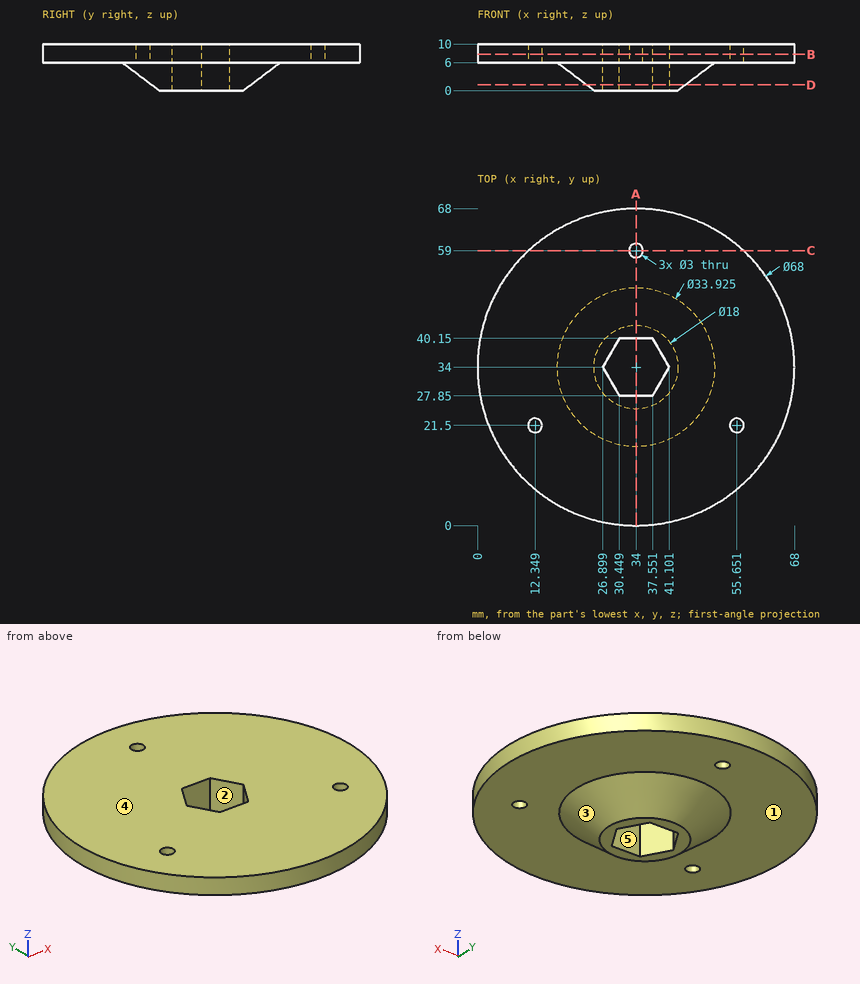
Could you check a few things on this drawing? It's one solid part, dimensions in mm from its lowest x, y, z. A direction names the side the tool comes from. Coordinates: 2 decimals unless noted, no trailing zeros. Order: outer loops, then holes, each group sorted by start corner. A loop starts at its lowest first (then second) coordinate and runs counter-clockwise, first axis right, second up. Notation, with made-up numbers: M 84,43 L 135,43 A13 ccw 135,62 Z; hole C -6.5,-4 d7. An arc over 180 degrees is marked long. Answer as CSV lines item,"result".
(1) I'm going to push flat-ended pins straight in: pin 1 (3.5 mm diameter, centred on x = 32.5, z = 4, fed in from -Y); pin 2 (5.5 mm diameter, centred on x = 34.5, z = 4, fed in from +Y); pin 3 (1 mm diameter, centred on x = 39.5, z = 2.5, fed in from +Y) (1 decimal). Where does each tip first touch, or does it pass through?
Geometry check:
pin 1,"y = 17.43"
pin 2,"y = 68"
pin 3,"y = 45.8"
(2) If we mould it in two halves opening along X, with no side actions, what happens to the marked faces 3, 4 and 5? For each: released by +X, released by -X, zero draft, split by the parting line, or undercut.
Geometry check:
face 3,"split by the parting line"
face 4,"zero draft"
face 5,"undercut"
(3) Suppose I cut it at B-B on z = 7.75. Please give me the cut outline in (x, y).
Geometry check:
outline,"C 34,34 d68; hole C 12.35,21.5 d3; hole M 26.9,34 L 30.45,27.85 L 37.55,27.85 L 41.1,34 L 37.55,40.15 L 30.45,40.15 Z; hole C 34,59 d3; hole C 55.65,21.5 d3"
(4) On a 3-axis mill with a long thin cutter (end or side, diameter ignored), from which of +Z, -Z, +X, -X, +Y, -Y can I reach the whole of each face in a straight line? I mean the marked faces 1 and 2. Say none if no direction works.
Geometry check:
face 1,"-Z"
face 2,"+Z, -Z"
(5) Suppose I cut it at A-A on x = 34. Please give me the cut outline in (y, z).
Geometry check:
outline,"M 0,6 L 17.04,6 L 25,0 L 27.85,0 L 27.85,10 L 0,10 Z; M 40.15,0 L 43,0 L 50.96,6 L 57.5,6 L 57.5,10 L 40.15,10 Z; M 60.5,6 L 68,6 L 68,10 L 60.5,10 Z"
(6) Suppose I cut it at D-D on z = 1.25. Please give me the cut outline in (x, y), plus the area to 3 significant figures.
Geometry check:
outline,"C 34,34 d21.32; hole M 26.9,34 L 30.45,27.85 L 37.55,27.85 L 41.1,34 L 37.55,40.15 L 30.45,40.15 Z"
area,"226 mm^2"
(7) Please list where these lines run through material, in increasing order: L1, parallel to Y at x = 34, z = 6.95; L2, parallel to Z at x = 24.5, y = 59.5; L3, parallel to Y at x = 41, z = 9.75 (1 decimal).
Geometry check:
L1,"0 to 27.85, 40.15 to 57.5, 60.5 to 68"
L2,"6 to 10"
L3,"0.7 to 33.8, 34.2 to 67.3"
(8) Suppose I cut it at C-C on y = 59. Please give me the cut outline in (x, z).
Geometry check:
outline,"M 10.96,6 L 32.5,6 L 32.5,10 L 10.96,10 Z; M 35.5,6 L 57.04,6 L 57.04,10 L 35.5,10 Z"
